Work out the finished part from the listing and answer in its coordinate system (mm). A direction names the side the tool comes from. Coordinates: 2 decimals unless noted, no trailing zeros. Order: outer loops, then holes, each group sorted by start corner. A loop starts at its lowest first (then second) coordinate and runs counter-clockwise, first axis right, second up. Notation, with made-up numbers: M 24,80 L 55,80 A18 ccw 55,86 Z; hole C -13,65.5 d6. An arc over 180 degrees is marked long. Answer in a Markdown table with one row per item. Add a question column.
Item 1: The part is cut by section C-C (x = 9). Write down the section's boundary in (y, z).
Item 2: Consider line 1 (Z direction, x = 24, y = 6.56); line 2 (Y direction, x = 1.5, z = 18.5); line 3 (Y direction, x = 26.5, z = -15) (3 decimals). Determine where each line is inside the solid, lowest interval first. Write a range as from..to.
Item 3: Flat-ended cylindrical pins translate along their axes: pin 1 Ø9 at (x, z) = (10, -27) entering from -Y; pin 2 Ø2 at (x, y) = (16.5, 80.5) entering from +Z; pin 3 Ø1 at (x, z) = (5.5, -62) entering from -Y. Find the tip coordinate at first contact, or state that the pin passes through.
Item 4: The part is cut by section D-D (z = 10). Write down the section's boundary in (x, y).
Item 5: The mould has two halves that part along Z. Classify faces 6 (the face through (10, 31.1, -15)), 7 (the face through (-4.535, 123.598, -14.16)), 8 (the face through (14, 113, -75)): released by +Z, released by -Z, zero draft, split by the parting line, or undercut.
Item 6: The part is cut by section A-A (y = 15.06). Write down the section's boundary in (x, z) (3 decimals).
Item 7: The part is cut by section B-B (z = -15). State how many separate pieces and enclosed holes the cut face has, then the cut area to 3 significant figures.
Item 8: Which of the six approach directions +Z, -Z, +X, -X, +Y, -Y give full straight-line access (tool end or side, diameter ignored) to faces 1 (the face through (22.1, 4.5, -13)), 2 (the face through (15, 93, -52)), 3 (the face through (20, 8, -20)), 4 (the face through (-6, 100, -14)), 5 (the face through (-4.465, 109.598, -14.16))?
Autodesk Inventor part; units mm, degrees
ref_plane "Work Plane1" through (0, 0, -15) normal (0, 0, 1) x (1, 0, 0)
ref_plane "YZ Plane" through (0, 0, 0) normal (1, 0, 0) x (0, 1, 0)
ref_plane "XZ Plane" through (0, 0, 0) normal (0, 1, 0) x (-1, 0, 0)
sketch "Sketch1" plane through (0, 0, 0) normal (0, 0, 1) x (1, 0, 0)
  line L0 (0, 0) -> (25, 0)
  line L1 (25, 0) -> (25, 40)
  line L2 (25, 40) -> (0, 40)
  line L3 (0, 40) -> (0, 0)
  dimension "d1" = 25
  dimension "d2" = 40
  dimension "d3" = 25
extrude "Extrusion1" add sketch "Sketch1" against normal blind 30
sketch "Sketch2" plane through (25, 0, 0) normal (1, 0, 0) x (0, 0, -1)
  line L0 (0, 0) -> (30, 0)
  circle A0 centre (15, 6.56) radius 2.46
extrude "Extrusion2" cut sketch "Sketch2" against normal blind 30
sketch "Sketch3" plane through (0, 0, 0) normal (-1, 0, 0) x (0, 0, 1)
  line L0 (0, 0) -> (-30, 0)
  line L1 (-25.05, 0) -> (-4.95, 0)
  line L2 (-4.95, 0) -> (-4.95, 33.12)
  line L3 (-4.95, 33.12) -> (-25.05, 33.12)
  line L4 (-25.05, 33.12) -> (-25.05, 0)
  dimension "d11" = 20.1
extrude "Extrusion3" cut sketch "Sketch3" against normal blind 20
sketch "Sketch4" plane through (0, 0, 0) normal (0, -1, 0) x (1, 0, 0)
  line L0 (20, -4.95) -> (20, -25.05)
  line L1 (20, -15) -> (25, -15)
  line L2 (25, 0) -> (25, -30)
  line L3 (20, -8.025) -> (25, -8.025)
  line L4 (25, -8.025) -> (25, -21.975)
  line L5 (25, -21.975) -> (20, -21.975)
  line L6 (20, -21.975) -> (20, -8.025)
  line L7 (20, -8.025) -> (25, -21.975) construction
  line L8 (25, -8.025) -> (20, -21.975) construction
  line L9 (25, -12.54) -> (25, -17.46)
  point P0 (0, 0)
  point P1 (22.5, -15)
  dimension "d14" = 13.95
extrude "Extrusion4" add sketch "Sketch4" along normal blind 15
sketch "Sketch5" plane through (20, 0, 0) normal (-1, 0, 0) x (0, 0, 1)
  circle A0 centre (-15, 6.56) radius 2.46
  circle A1 centre (-15, 6.56) radius 4.7025
  circle A2 centre (-15, 6.56) radius 2.46
  circle A3 centre (-15, 6.56) radius 2.46
  point P0 (0, 0)
  dimension "d17" = 9.405
extrude "Extrusion5" cut sketch "Sketch5" against normal blind 2.1
sketch "Sketch6" plane through (25, 0, 0) normal (1, 0, 0) x (0, 0, -1)
  circle A0 centre (15, 6.56) radius 4.7025
  line L0 (15, 6.56) -> (15, 23.56)
  circle A1 centre (15, 23.56) radius 2.46
  point P0 (0, 0)
  dimension "d20" = 17
  dimension "d21" = 4.92
extrude "Extrusion6" cut sketch "Sketch6" against normal blind 10 contours A1
sketch "Sketch7" plane through (20, 0, 0) normal (-1, 0, 0) x (0, 0, 1)
  circle A0 centre (-15, 23.56) radius 2.46
  circle A1 centre (-15, 23.56) radius 4.7025
  point P0 (0, 0)
  dimension "d24" = 9.405
extrude "Extrusion7" cut sketch "Sketch7" against normal blind 2.1
sketch "Sketch9" plane through (25, 0, 0) normal (1, 0, 0) x (0, 0, -1)
  circle A0 centre (15, 6.56) radius 2.46
  circle A1 centre (15, 6.56) radius 2.46
  circle A2 centre (15, 23.56) radius 2.46
  circle A3 centre (15, 23.56) radius 2.46
  line L0 (30, 40) -> (30, 0)
  line L1 (30, 0) -> (30, 40)
  line L2 (30, 40) -> (0, 40)
  line L3 (0, 40) -> (0, 0)
  line L4 (0, 0) -> (8.025, 0)
  line L5 (21.975, 0) -> (21.975, -15)
  line L6 (21.975, -15) -> (8.025, -15)
  line L7 (8.025, -15) -> (8.025, 0)
  line L8 (0, 0) -> (8.025, 0)
  line L9 (21.975, 0) -> (30, 0)
extrude "Extrusion8" add sketch "Sketch9" along normal blind 5
sketch "Sketch10" plane through (0, 40, 0) normal (0, 1, 0) x (1, 0, 0)
  line L0 (0, 30) -> (30, 30)
  line L1 (30, 0) -> (0, 0)
  line L2 (0, 30) -> (30, 30)
  line L3 (30, 30) -> (30, 0)
  line L4 (30, 0) -> (0, 0)
  line L5 (0, 0) -> (0, 30)
extrude "Extrusion9" add sketch "Sketch10" along normal blind 30
sketch "Sketch12" plane through (30, 0, 0) normal (1, 0, 0) x (0, 0, -1)
  circle A0 centre (15, 6.56) radius 2.46
  line L0 (15, 6.56) -> (15, 15.06)
  circle A1 centre (15, 15.06) radius 2.525
  point P0 (0, 0)
  dimension "d31" = 8.5
  dimension "d33" = 5.05
extrude "Extrusion10" cut sketch "Sketch12" against normal blind 30 contours A1
sketch "Sketch14" plane through (0, 0, 0) normal (0, 0, 1) x (1, 0, 0)
  line L0 (30, 70) -> (0, 70)
  line L1 (0, 70) -> (0, 85)
  line L2 (30, 0) -> (30, 70)
  line L3 (30, 118) -> (30, 70)
  line L4 (30, 105) -> (30, 100)
  line L5 (-12, 133) -> (15, 133)
  line L6 (-7, 130.5) -> (-12, 133)
  line L7 (-7, 130.5) -> (-2, 116.5)
  line L8 (-7, 102.5) -> (-12, 100)
  line L9 (-7, 102.5) -> (-2, 116.5)
  line L10 (30, 118) -> (15, 133)
  line L11 (0, 100) -> (-12, 100)
  line L12 (0, 100) -> (0, 85)
  point P0 (0, 0)
  dimension "d79" = 12
extrude "Extrusion12" add sketch "Sketch14" against normal blind 30
sketch "Sketch15" plane through (0, 0, -25.05) normal (-1, 0, 0) x (0, 0, 1)
  line L0 (0, 33.12) -> (20.1, 33.12)
  line L1 (20.1, 33.12) -> (20.1, 0)
  line L2 (0, 33.12) -> (20.1, 33.12)
  line L3 (20.1, 33.12) -> (20.1, 31.1)
  line L4 (20.1, 31.1) -> (0, 31.1)
  line L5 (0, 31.1) -> (0, 33.12)
  point P0 (25.05, 0)
  dimension "d57" = 2.02
extrude "Extrusion13" add sketch "Sketch15" against normal blind 20
sketch "Sketch22" plane through (0, 0, 0) normal (0, 0, 1) x (1, 0, 0)
  line L0 (0, 100) -> (-12, 100)
  line L1 (0, 100) -> (-12, 100)
  line L2 (-12, 100) -> (-7, 102.5)
  line L3 (-12, 100) -> (-7, 102.5)
  line L4 (-7, 102.5) -> (-2, 116.5)
  line L5 (-7, 102.5) -> (-2, 116.5)
  line L6 (-2, 116.5) -> (-7, 130.5)
  line L7 (-2, 116.5) -> (-7, 130.5)
  line L8 (-7, 130.5) -> (-12, 133)
  line L9 (-7, 130.5) -> (-12, 133)
  line L10 (-12, 133) -> (15, 133)
  line L11 (-12, 133) -> (15, 133)
  line L12 (15, 133) -> (30, 118)
  line L13 (15, 133) -> (30, 118)
  line L14 (30, 118) -> (30, 93)
  line L15 (30, 0) -> (30, 118)
  line L16 (30, 93) -> (0, 93)
  line L17 (0, 100) -> (0, 0)
  line L18 (0, 93) -> (0, 100)
  dimension "d80" = 25
extrude "Extrusion14" add sketch "Sketch22" along normal blind 45
ref_plane "Work Plane1" through (0, 0, -15) normal (0, 0, 1) x (1, 0, 0)
mirror "Mirror1" about plane through (0, 0, -15) normal (0, 0, 1) of "Extrusion14"
properties part number "rec_b_28mm_x_120mm"
Reply:
| question | item | result |
|---|---|---|
| 1 | outline | M 0,-30 L 93,-30 L 93,-75 L 133,-75 L 133,45 L 93,45 L 93,0 L 0,0 L 0,-4.95 L 31.1,-4.95 L 31.1,-25.05 L 0,-25.05 Z |
| 2 | line 1 | z = -30..-17.46, -12.54..0 |
| 2 | line 2 | y = 93..133 |
| 2 | line 3 | y = -15..4.1, 9.02..12.535, 17.585..21.1, 26.02..121.5 |
| 3 | pin 1 | stops at y = 0 |
| 3 | pin 2 | stops at z = 0 |
| 3 | pin 3 | stops at y = 93 |
| 4 | outline | M -12,100 L 0,100 L 0,93 L 30,93 L 30,118 L 15,133 L -12,133 L -7,130.5 L -2,116.5 L -7,102.5 Z |
| 5 | face 6 | undercut |
| 5 | face 7 | zero draft |
| 5 | face 8 | released by -Z |
| 6 | outline | M 0,-30 L 30,-30 L 30,-17.525 L 20,-17.525 L 20,-25.05 L 0,-25.05 Z; M 0,-4.95 L 20,-4.95 L 20,-12.475 L 30,-12.475 L 30,0 L 0,0 Z |
| 7 | separate pieces | 4 |
| 7 | enclosed holes | 0 |
| 7 | area | 3,410 mm2 |
| 8 | face 1 | -X |
| 8 | face 2 | -Z, +X, -X, -Y |
| 8 | face 3 | -X, -Y |
| 8 | face 4 | +Z, -Z, -X, -Y |
| 8 | face 5 | +Z, -Z, -X |
